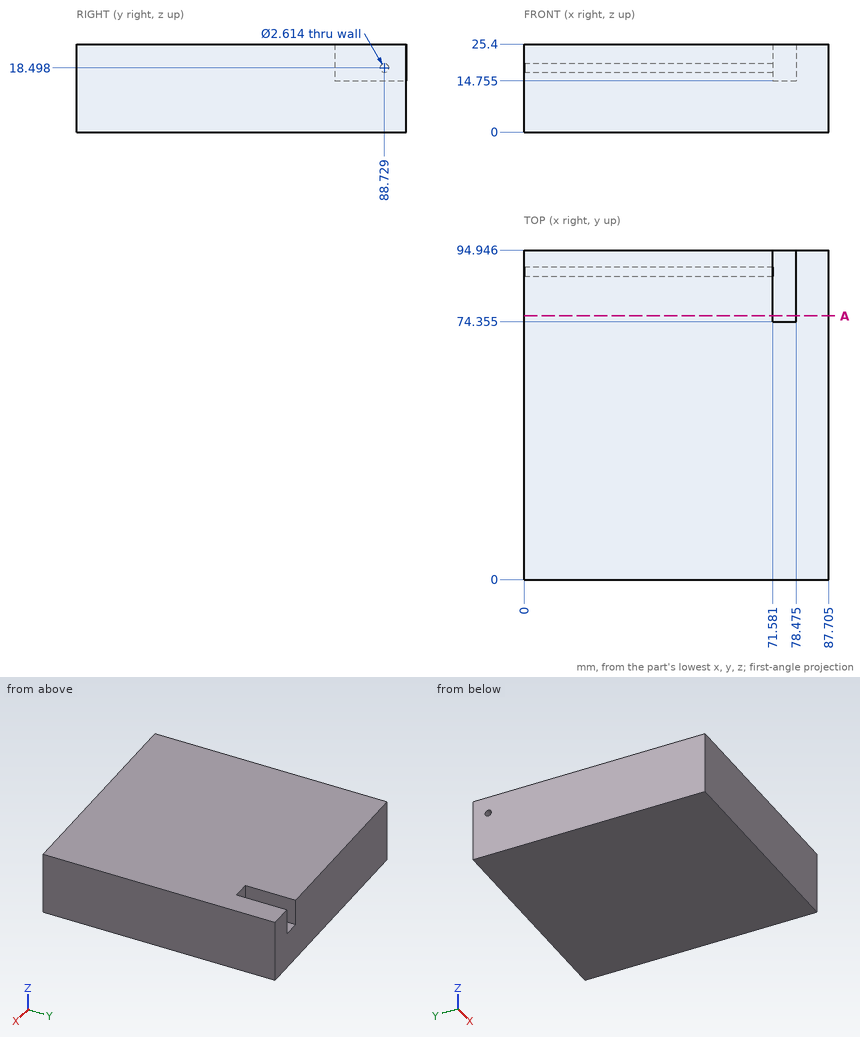
Print and shaded views of the part. All mm, measured from the part's lowest x, y and z. Round coordinates to 2 decimals unless told otherwise and drop trailing zeros. Write each loop counter-clockwise with the first axis right and the second up, starting at its lowest first coordinate (ties: lowest second). Pieces come first, ordered by that corner, then holes. Notation, with made-up numbers: (82, -5) -> (122, -5) arc R17 ccw to (122, 23) -> close; hole circle Ø9 at (20.25, -24.5). An arc over 180 degrees is marked (long way). Answer in a Markdown table with one row per item. Add a question column.
Item 1: Drop flat-ended pins along their axis: pin 1 Ø5.5 at (y, z) = (80.5, 18) entering from -X; pin 2 Ø5.5 at (x, y) = (75, 85.5) entering from +Z (1 decimal). Give the stop position or say it passes through.
Item 2: Drill centre lines: line 1 (X direction, y = 85.5, z = 19) (1 decimal); line 2 (Z direction, x = 31, y = 89). Where is each one in solid material? Low to high. Write a range as from..to.
Item 3: Saw through at A-A, the plane y = 76. Write the cut outline in (x, z) (1 decimal).
Findings below:
| question | item | result |
|---|---|---|
| 1 | pin 1 | stops at x = 0 |
| 1 | pin 2 | stops at z = 14.8 |
| 2 | line 1 | x = 0..71.6, 78.5..87.7 |
| 2 | line 2 | z = 0..17.22, 19.78..25.4 |
| 3 | outline | (0, 0) -> (87.7, 0) -> (87.7, 25.4) -> (78.5, 25.4) -> (78.5, 14.8) -> (71.6, 14.8) -> (71.6, 25.4) -> (0, 25.4) -> close |
